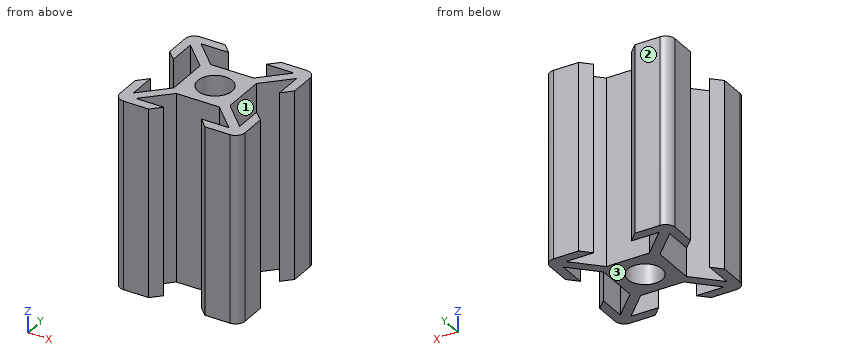
```python
from build123d import *

# Parameters (mm, degrees)
SKETCH_R  = 2.75
PAD_DEPTH = 30


with BuildPart() as part:
    # Sketch → Pad (new body)
    with BuildSketch(Plane.XY):
        with BuildLine():
            ThreePointArc((-8.5, 10), (-9.56066, 9.56066), (-10, 8.5))
            Line((-10, 8.5), (-10, 4.5))
            Line((-10, 4.5), (-8.5, 3))
            Line((-8.5, 3), (-8.5, 7.43934))
            Line((-8.5, 7.43934), (-4.5, 3.43934))
            Line((-4.5, 3.43934), (-4.5, -3.43934))
            Line((-4.5, -3.43934), (-8.5, -7.43934))
            Line((-8.5, -7.43934), (-8.5, -3))
            Line((-8.5, -3), (-10, -4.5))
            Line((-10, -4.5), (-10, -8.5))
            ThreePointArc((-10, -8.5), (-9.56066, -9.56066), (-8.5, -10))
            Line((-8.5, -10), (-4.5, -10))
            Line((-4.5, -10), (-3, -8.5))
            Line((-3, -8.5), (-7.43934, -8.5))
            Line((-7.43934, -8.5), (-3.43934, -4.5))
            Line((-3.43934, -4.5), (3.43934, -4.5))
            Line((3.43934, -4.5), (7.43934, -8.5))
            Line((7.43934, -8.5), (3, -8.5))
            Line((3, -8.5), (4.5, -10))
            Line((4.5, -10), (8.5, -10))
            ThreePointArc((8.5, -10), (9.56066, -9.56066), (10, -8.5))
            Line((10, -8.5), (10, -4.5))
            Line((10, -4.5), (8.5, -3))
            Line((8.5, -3), (8.5, -7.43934))
            Line((8.5, -7.43934), (4.5, -3.43934))
            Line((4.5, -3.43934), (4.5, 3.43934))
            Line((4.5, 3.43934), (8.5, 7.43934))
            Line((8.5, 7.43934), (8.5, 3))
            Line((8.5, 3), (10, 4.5))
            Line((10, 4.5), (10, 8.5))
            ThreePointArc((10, 8.5), (9.56066, 9.56066), (8.5, 10))
            Line((8.5, 10), (4.5, 10))
            Line((4.5, 10), (3, 8.5))
            Line((3, 8.5), (7.43934, 8.5))
            Line((7.43934, 8.5), (3.43934, 4.5))
            Line((-3.43934, 4.5), (3.43934, 4.5))
            Line((-7.43934, 8.5), (-3.43934, 4.5))
            Line((-3, 8.5), (-7.43934, 8.5))
            Line((-4.5, 10), (-3, 8.5))
            Line((-8.5, 10), (-4.5, 10))
        make_face()
        Circle(SKETCH_R, mode=Mode.SUBTRACT)
    extrude(amount=PAD_DEPTH)


solid = part.part
```
CAD build for the part. Positions are in the model's coordinates, mm. Face numbers are marked on the shaded views. Round coordinates to 2 decimals unless told otherwise and drop trailing zeros. Write each loop counter-clockwise with the first axis right and the second up, starting at its lowest first coordinate (ties: lowest second). Pieces come first, ordered by that corner, then holes.
Item 1: Band-saw the part on D-D on y = -5.5. Write the cut outline in (x, z), then the cut area to 3 significant figures.
Filled in:
outline: (-10, 0) - (-8.5, 0) - (-8.5, 30) - (-10, 30) - close; (-6.56, 0) - (-4.44, 0) - (-4.44, 30) - (-6.56, 30) - close; (4.44, 0) - (6.56, 0) - (6.56, 30) - (4.44, 30) - close; (8.5, 0) - (10, 0) - (10, 30) - (8.5, 30) - close
area: 217 mm2
Item 2: Band-saw the part on C-C on x = -5.25. Write the cut outline in (y, z).
Filled in:
outline: (-10, 0) - (-8.5, 0) - (-8.5, 30) - (-10, 30) - close; (-6.31, 0) - (-4.19, 0) - (-4.19, 30) - (-6.31, 30) - close; (4.19, 0) - (6.31, 0) - (6.31, 30) - (4.19, 30) - close; (8.5, 0) - (10, 0) - (10, 30) - (8.5, 30) - close
Item 3: Drill centre lines: L1, parallel to Y at x = 0, z = 8.5; L2, parallel to Y at x = -5, z = 10; L3, parallel to Y at x = 4, z = 12. Where is each one in solid material? Low to high.
Filled in:
L1: y = -4.5 to -2.75, 2.75 to 4.5
L2: y = -10 to -8.5, -6.06 to -3.94, 3.94 to 6.06, 8.5 to 10
L3: y = -9.5 to -8.5, -5.06 to 5.06, 8.5 to 9.5
Item 4: Mould opens along Y. For the marked faces 1, 2 and 3 say: released by +Y, released by -Y, zero draft, split by the parting line, or undercut.
Filled in:
face 1: undercut
face 2: released by +Y
face 3: zero draft
Item 5: Drop flat-ended pins along their axis: pin 1 Ø2 at (x, z) = (-0.5, 8) entering from -Y; pin 2 Ø3 at (x, y) = (-1, 0) entering from -Z; pin 3 Ø5.5 at (y, z) = (-0.5, 10.5) entering from -X; pin 4 Ø7.5 at (y, z) = (-0.5, 22) entering from +X. Give the stop position or say it passes through.
Filled in:
pin 1: stops at y = -4.5
pin 2: passes through
pin 3: stops at x = -8.75
pin 4: stops at x = 9.75
Item 6: Band-saw the part on A-A on x = 0. Write the cut outline in (y, z).
Filled in:
outline: (-4.5, 0) - (-2.75, 0) - (-2.75, 30) - (-4.5, 30) - close; (2.75, 0) - (4.5, 0) - (4.5, 30) - (2.75, 30) - close
